from build123d import *

# Parameters (mm, degrees)
BOSS_EXTRUDE1_DEPTH = 37
SKETCH2_R           = 1.75
CUT_EXTRUDE1_DEPTH  = 6


with BuildPart() as part:
    # Sketch1 → Boss-Extrude1 (new body)
    with BuildSketch(Plane.XY):
        Polygon((1, 11.5), (35, 11.5), (35, -1), (44, -1), (44, 0), (36, 0), (36, 12.5), (0, 12.5), (0, 0), (-8, 0), (-8, -1), (1, -1), align=None)
    extrude(amount=BOSS_EXTRUDE1_DEPTH)

    # Sketch2 → Cut-Extrude1 (cut)
    with BuildSketch(Plane(origin=(0, 0, 0), x_dir=(1, 0, 0), z_dir=(0, 1, 0))):
        with Locations((-4, -27)):
            Circle(SKETCH2_R)
        with Locations((-4, -10)):
            Circle(SKETCH2_R)
        with Locations((40, -27)):
            Circle(SKETCH2_R)
        with Locations((40, -10)):
            Circle(SKETCH2_R)
    extrude(amount=-CUT_EXTRUDE1_DEPTH, mode=Mode.SUBTRACT)


solid = part.part
CAD build for the part. Positions are in the model's coordinates, mm. A direction names the side the tool comes from. Coordinates: 2 decimals unless noted, no trailing zeros. Write each loop counter-clockwise with the first axis right and the second up, starting at its lowest first coordinate (ties: lowest second). Pieces come first, ordered by that corner, then holes. Notation, with made-up numbers: (19, -5.75) - (58, -5.75) arc R28 cw to (58, 18.25) - close; hole circle Ø8 at (60.5, 11). An arc over 180 degrees is marked (long way). Use a Markdown table: item, result. Add a question column.
Item 1: Band-saw the part on A-A, the plane x = 40. Give the cut face in (y, z), and give its area (3 significant figures).
Item 2: Band-saw the part on D-D, the plane z = 20. Give the cut face in (x, y), and give its area (3 significant figures).
Item 3: Band-saw the part on C-C, the plane y = 4. Give the cut face in (x, z).
Item 4: Flat gauge pins, fed straight in: pin 1 (4 mm diameter, centred on y = 6.5, z = 26.5, fed in from -X); pin 2 (2 mm diameter, centred on x = 22.5, z = 30.5, fed in from -Y); pin 3 (4.5 mm diameter, centred on x = 40, z = 27, fed in from +Y). Where does each tip first touch, or does it go through?
Item 5: Drill centre lines: L1, parallel to X at y = -0.55, z = 10; L2, parallel to Z at x = 40, y = -0.45; L3, parallel to X at y = 1.75, z = 19.5. Where is each one in solid material? Low to high. Write a range as from..to.
Item 6: Band-saw the part on B-B, the plane z = 10. Give the cut face in (x, y).
Item 7: 3-axis set-ups, long thin cutter, end or side, ignore diameter. For faces 1 (the face through (36, 6, 18)), 2 (the face through (-4, 0, 18)), 3 (the face through (39, -1, 18)), 4 (the face through (35, 5, 18)): which of +Z, -Z, +X, -X, +Y, -Y reach the whole face in a straight line?
Item 8: Mould opens along Z. For faces 5 (the face through (18, 11.5, 18)), 6 (the face through (41.669, -0.493, 9.474)), 7 (the face through (16, 12, 0)) say: pulls with the +Z half, pulls with the -Z half, needs draft (parallel to the pull), parting line crosses it, or undercut.
Numbers:
| question | item | result |
|---|---|---|
| 1 | outline | (-1, 0) - (0, 0) - (0, 8.25) - (-1, 8.25) - close; (-1, 11.75) - (0, 11.75) - (0, 25.25) - (-1, 25.25) - close; (-1, 28.75) - (0, 28.75) - (0, 37) - (-1, 37) - close |
| 1 | area | 30.0 mm2 |
| 2 | outline | (-8, -1) - (1, -1) - (1, 11.5) - (35, 11.5) - (35, -1) - (44, -1) - (44, 0) - (36, 0) - (36, 12.5) - (0, 12.5) - (0, 0) - (-8, 0) - close |
| 2 | area | 77.0 mm2 |
| 3 | outline | (0, 0) - (1, 0) - (1, 37) - (0, 37) - close; (35, 0) - (36, 0) - (36, 37) - (35, 37) - close |
| 4 | pin 1 | x = 0 |
| 4 | pin 2 | y = 11.5 |
| 4 | pin 3 | y = 0 |
| 5 | L1 | -8..-5.75, -2.25..1, 35..38.25, 41.75..44 |
| 5 | L2 | 0..8.25, 11.75..25.25, 28.75..37 |
| 5 | L3 | 0..1, 35..36 |
| 6 | outline | (-8, -1) - (-5.75, -1) - (-5.75, 0) - (-8, 0) - close; (-2.25, -1) - (1, -1) - (1, 11.5) - (35, 11.5) - (35, -1) - (38.25, -1) - (38.25, 0) - (36, 0) - (36, 12.5) - (0, 12.5) - (0, 0) - (-2.25, 0) - close; (41.75, -1) - (44, -1) - (44, 0) - (41.75, 0) - close |
| 7 | face 1 | +Z, -Z, +X, +Y |
| 7 | face 2 | +Z, -Z, -X, +Y |
| 7 | face 3 | +Z, -Z, +X, -X, -Y |
| 7 | face 4 | +Z, -Z, -Y |
| 8 | face 5 | needs draft |
| 8 | face 6 | undercut |
| 8 | face 7 | pulls with the -Z half |
